Can you work these out from the drawing? Everything is in mm from the part's minimum corner. Round coordinates to 2 decimals unless told otherwise and drop trailing zeros. Loops run counter-clockwise (first coordinate to the right, second up) from the corner with the lowest first, then second, coordinate; pieces in that order, holes last. Notation, with made-up numbers: M -38.5,1.5 L -4.5,1.5 A16 cw -4.5,11.5 Z; hole C 65,-5 d5. An arc over 180 degrees is marked long. Answer in a Markdown table with one row per item.
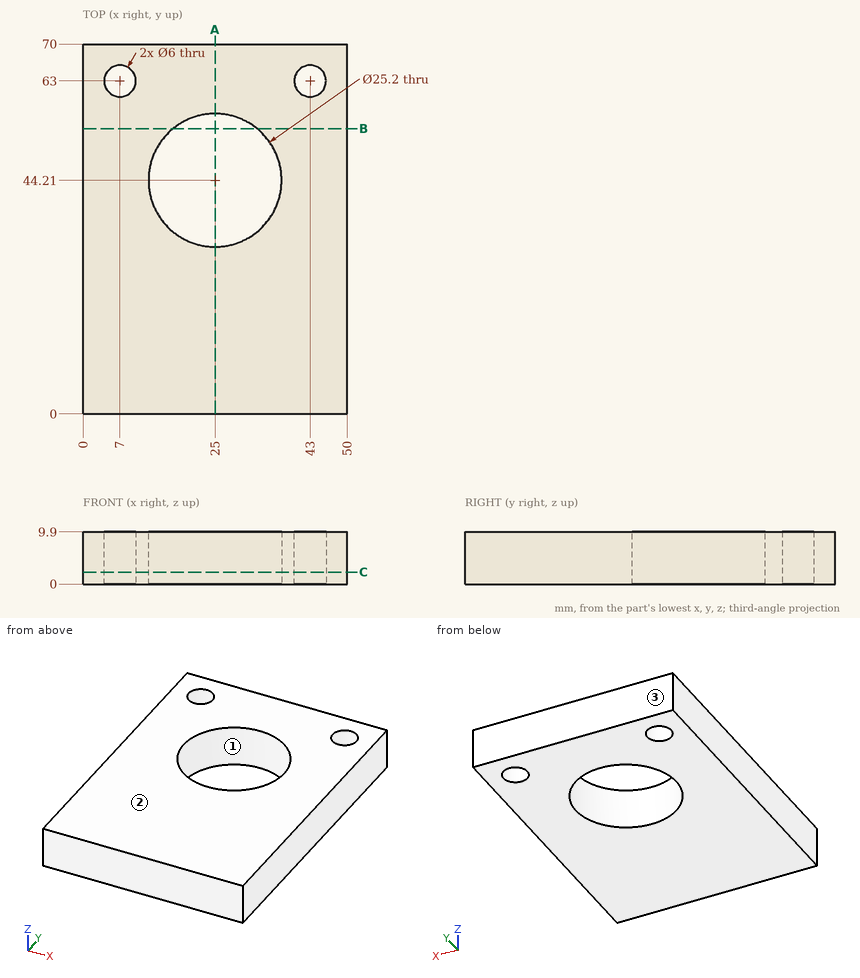
1) I want a section at C-C, the plane z = 2.25. Please give me the cut outline in (x, y).
Computed:
| item | result |
|---|---|
| outline | M 0,0 L 50,0 L 50,70 L 0,70 Z; hole C 7,63 d6; hole C 25,44.21 d25.2; hole C 43,63 d6 |
2) I want a section at A-A, the plane x = 25. Please give me the cut outline in (y, z).
Computed:
| item | result |
|---|---|
| outline | M 0,0 L 31.61,0 L 31.61,9.9 L 0,9.9 Z; M 56.81,0 L 70,0 L 70,9.9 L 56.81,9.9 Z |
3) I need wall thicknesses on line 1 (X direction, y = 63, z = 6); line 2 (Y direction, x = 25, z = 9); line 3 (Y direction, x = 43, z = 7.5). Which ranges of each line are inside material? Lowest first, please.
Computed:
| item | result |
|---|---|
| line 1 | x = 0 to 4, 10 to 40, 46 to 50 |
| line 2 | y = 0 to 31.61, 56.81 to 70 |
| line 3 | y = 0 to 60, 66 to 70 |
4) I want a section at B-B, the plane y = 54. Please give me the cut outline in (x, z), plus the area to 3 significant figures.
Computed:
| item | result |
|---|---|
| outline | M 0,0 L 17.07,0 L 17.07,9.9 L 0,9.9 Z; M 32.93,0 L 50,0 L 50,9.9 L 32.93,9.9 Z |
| area | 338 mm² |
5) If we mould it in two halves opening along Y, with no side actions, what happens to the marked faces 1, 2 and 3? For each: released by +Y, released by -Y, zero draft, split by the parting line, or undercut.
Computed:
| item | result |
|---|---|
| face 1 | undercut |
| face 2 | zero draft |
| face 3 | released by +Y |
